Read the model definition and answer for the solid it produces. Units are mm, in the model's axes. A direction names the side the tool comes from. Coordinates: 2 decimals unless noted, no trailing zeros. Write each loop counter-clockwise with the first axis right and the second up, starting at its lowest first coordinate (ties: lowest second). Pieces come first, ordered by that corner, then holes.
1) Which of the six approach directions +Z, -Z, +X, -X, +Y, -Y give full straight-line access (tool end or side, diameter ignored) to faces 1 (the face through (0, 1, 4.5)), 2 (the face through (0, 2, -5))?
2) The part is cut by section C-C (z = 0). Determine the outline of the cut face in (x, y).
3) The part is cut by section A-A (z = 14.6). Determine the outline of the cut face in (x, y).
4) The part is cut by section D-D (x = 1.5). Determine the outline of the cut face in (y, z), then the cut area to 3 significant figures.
5) Each of these flat-tipped pins is pushed along its axis until it touches: pin 1 Ø4 at (x, z) = (-14.6, 14.6) entering from +Y; pin 2 Ø0.6 at (x, y) = (-2.5, 1.5) entering from +Z; pin 3 Ø2.5 at (x, z) = (14.6, -14.6) entering from -Y; pin 4 Ø1 at (x, y) = (12.5, 1.5) entering from +Z. Where does it stop, or does it pass through?
6) The part is cut by section B-B (y = 0.8). Determine the outline of the cut face in (x, z).
7) Find the intervals of material crossed by line 1 (X direction, y = 1.8, z = 14.6); line 2 (Z direction, x = -0.5, y = 1.3), in increasing order.
8) Determine the mould class of faces 3 (the face through (-10.9, 1, 0.4)), 4 (the face through (0, 0, -5)), 5 (the face through (5.506, 0.986, 24.796)) for opening direction X: +X half, -X half, draft (parallel to the pull), parting line (faces both ways), or undercut.
Autodesk Inventor part; units mm, degrees
ref_plane "YZ Plane" through (0, 0, 0) normal (1, 0, 0) x (0, 1, 0)
ref_plane "XZ Plane" through (0, 0, 0) normal (0, 1, 0) x (-1, 0, 0)
ref_plane "XY Plane" through (0, 0, 0) normal (0, 0, 1) x (1, 0, 0)
sketch "Skizze1" plane through (0, 0, 0) normal (0, 1, 0) x (-1, 0, 0)
  circle A0 centre (0, 0) radius 25.4
  dimension "d0" = 50.8
extrude "Extrusion1" add sketch "Skizze1" along normal blind 2
sketch "Skizze2" plane through (0, 0, 0) normal (0, -1, 0) x (1, 0, 0)
  circle A0 centre (0, 0) radius 25.4
  line L0 (-14.6, 14.6) -> (14.6, 14.6) construction
  line L1 (14.6, 14.6) -> (14.6, -14.6) construction
  line L2 (14.6, -14.6) -> (-14.6, -14.6) construction
  line L3 (-14.6, -14.6) -> (-14.6, 14.6) construction
  line L4 (0, 0) -> (14.6, 0) construction
  line L5 (0, 0) -> (0, 14.6) construction
  dimension "d3" = 29.2
  dimension "d4" = 29.2
hole "Bohrung1" at (-14.6, 0, 14.6) at (14.6, 0, 14.6) at (14.6, 0, -14.6) at (-14.6, 0, -14.6) direction (0, 1, 0) diameter 3 end through all countersink diameter 6 countersink angle 90
sketch "Skizze7" plane through (0, 0, 0) normal (0, -1, 0) x (1, 0, 0)
  circle A0 centre (0, 0) radius 25.4
  line L0 (-8.75, 4.5) -> (8.75, 4.5)
  line L1 (8.75, 4.5) -> (8.75, -4.5)
  line L2 (8.75, -4.5) -> (-8.75, -4.5)
  line L3 (-8.75, -4.5) -> (-8.75, 4.5)
  line L4 (0, 0) -> (8.75, 0) construction
  line L5 (0, 0) -> (0, 4.5) construction
  line L6 (0, 0) -> (12.5, 0) construction
  line L7 (0, 0) -> (-12.5, 0) construction
  dimension "d25" = 17.5
  dimension "d26" = 9
  dimension "d28" = 12.5
  dimension "d29" = 12.5
extrude "Extrusion5" cut sketch "Skizze7" against normal blind 2 contours L0 L1 L2 L3
sketch "Skizze8" plane through (0, 0, 0) normal (0, -1, 0) x (1, 0, 0)
  circle A0 centre (0, 0) radius 25.4
  line L0 (0, 0) -> (12.5, 0) construction
  line L1 (0, 0) -> (-12.5, 0) construction
  dimension "d32" = 12.5
  dimension "d33" = 12.5
hole "Bohrung2" at (-12.5, 0, 0) at (12.5, 0, 0) direction (0, 1, 0) diameter 3.3 end through all
properties part number "anschluss_daten"
Reported:
1. face 1: +Y, -Y
1. face 2: +Z, -Z, +X, -X, +Y
2. outline: (-25.4, 0) - (-14.15, 0) - (-14.15, 2) - (-25.4, 2) - close; (-10.85, 0) - (-8.75, 0) - (-8.75, 2) - (-10.85, 2) - close; (8.75, 0) - (10.85, 0) - (10.85, 2) - (8.75, 2) - close; (14.15, 0) - (25.4, 0) - (25.4, 2) - (14.15, 2) - close
3. outline: (-20.78, 0) - (-17.6, 0) - (-16.1, 1.5) - (-16.1, 2) - (-20.78, 2) - close; (-13.1, 1.5) - (-11.6, 0) - (11.6, 0) - (13.1, 1.5) - (13.1, 2) - (-13.1, 2) - close; (16.1, 1.5) - (17.6, 0) - (20.78, 0) - (20.78, 2) - (16.1, 2) - close
4. outline: (0, -25.36) - (2, -25.36) - (2, -4.5) - (0, -4.5) - close; (0, 4.5) - (2, 4.5) - (2, 25.36) - (0, 25.36) - close
4. area: 83.4 mm2
5. pin 1: stops at y = 2
5. pin 2: stops at z = 25.3
5. pin 3: passes through
5. pin 4: stops at z = 22.39
6. outline: circle Ø50.8 at (0, 0); hole circle Ø4.4 at (-14.6, -14.6); hole circle Ø4.4 at (-14.6, 14.6); hole circle Ø3.3 at (-12.5, 0); hole (-8.75, -4.5) - (8.75, -4.5) - (8.75, 4.5) - (-8.75, 4.5) - close; hole circle Ø3.3 at (12.5, 0); hole circle Ø4.4 at (14.6, -14.6); hole circle Ø4.4 at (14.6, 14.6)
7. line 1: x = -20.78 to -16.1, -13.1 to 13.1, 16.1 to 20.78
7. line 2: z = -25.4 to -4.5, 4.5 to 25.4
8. face 3: undercut
8. face 4: draft
8. face 5: parting line
